For this review, take the finished solid that the model builds, in its own axes (mm). Face numbers are marked on the shaded views. A direction names the side the tool comes from. Round coordinates to 2 decimals unless told otherwise and drop trailing zeros. Order: outer loops, then holes, each group sorted by start corner. A loop starts at its lowest first (then second) coordinate and runs counter-clockwise, first axis right, second up. Notation, with made-up numbers: (-32.5, 36) -> (-3.5, 36) arc R20 ccw to (-3.5, 40) -> close; hole circle Ø4 at (-0.5, 70). An arc over 180 degrees is marked (long way). Answer in a Markdown table with one row per item.
```python
from build123d import *

# Parameters (mm, degrees)
F0_R     = 12.7
F0_R_2   = 6
F0_R_3   = 3.025
F1_DEPTH = 5
F2_DEPTH = 9
F3_D     = 2.4
F6_D     = 2.4
F6_DEPTH = 10
F6_TIP   = 0.7210327428


with BuildPart() as f1:
    # F0 (on Front) → F1 (new body)
    with BuildSketch(Plane.XZ):
        Circle(F0_R)
        Circle(F0_R_2, mode=Mode.SUBTRACT)
        Circle(F0_R_2)
        Circle(F0_R_3, mode=Mode.SUBTRACT)
    extrude(amount=F1_DEPTH)

    # F0 (on Front) → F2 (join)
    with BuildSketch(Plane.XZ):
        Circle(F0_R_2)
        Circle(F0_R_3, mode=Mode.SUBTRACT)
    extrude(amount=F2_DEPTH)

    # F3 (through all)
    with Locations(Plane(origin=(0, 0, 0), x_dir=(1, 0, 0), z_dir=(0, 1, 0))):
        with Locations((9.5, 0), (4.75, -8.227241336), (-4.75, -8.227241336), (-9.5, 0), (-4.75, 8.227241336), (4.75, 8.227241336)):
            Hole(F3_D / 2)

    # F6
    with Locations(Plane.XY.offset(12.7)):
        with Locations((0, -2.5), (0, -7)):
            Hole(F6_D / 2, depth=F6_DEPTH)
            with Locations((0, 0, -(F6_DEPTH + F6_TIP / 2))):  # 118° drill point
                Cone(0, F6_D / 2, F6_TIP, mode=Mode.SUBTRACT)


solid = f1.part
```
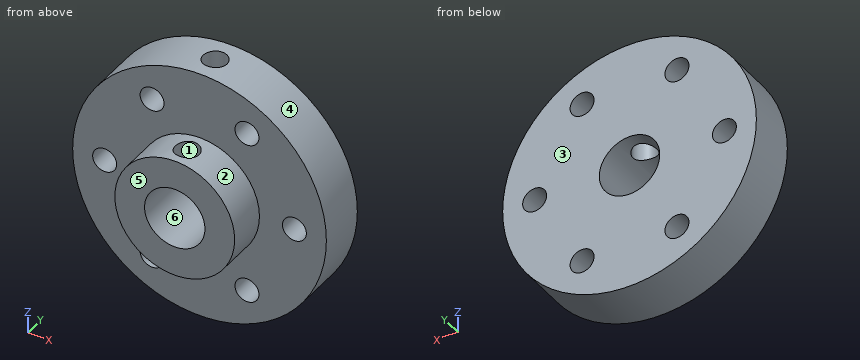
Q1. Take a section at C-C, the plane y = -1.75. Write out the cut boundary in (x, z) (3 decimals).
Answer key:
| item | result |
|---|---|
| outline | (-0.937, 2.876) -> (-0.937, 12.665) arc R12.7 ccw (long way) to (0.937, 12.665) -> (0.937, 2.876) arc R3.025 cw (long way) to start; hole circle Ø2.4 at (-9.5, 0); hole circle Ø2.4 at (-4.75, -8.227); hole circle Ø2.4 at (-4.75, 8.227); hole circle Ø2.4 at (4.75, -8.227); hole circle Ø2.4 at (4.75, 8.227); hole circle Ø2.4 at (9.5, 0) |
Q2. Take a section at D-D, the plane x = -4.25. Write out the cut boundary in (y, z), then the cut area to 3 significant figures.
Answer key:
| item | result |
|---|---|
| outline | (-9, -4.24) -> (-5, -4.24) -> (-5, -7.14) -> (0, -7.14) -> (0, 7.14) -> (-5, 7.14) -> (-5, 4.24) -> (-9, 4.24) -> close; (-5, -11.97) -> (0, -11.97) -> (0, -9.32) -> (-5, -9.32) -> close; (-5, 9.32) -> (0, 9.32) -> (0, 11.97) -> (-5, 11.97) -> close |
| area | 132 mm^2 |
Q3. Take a section at A-A, the plane x = 0. Write out the cut boundary in (y, z) (3 decimals).
Answer key:
| item | result |
|---|---|
| outline | (-9, -6) -> (-5, -6) -> (-5, -12.7) -> (0, -12.7) -> (0, -3.025) -> (-9, -3.025) -> close; (-9, 3.025) -> (-8.2, 3.025) -> (-8.2, 6) -> (-9, 6) -> close; (-5.8, 3.025) -> (-3.7, 3.025) -> (-3.7, 12.7) -> (-5, 12.7) -> (-5, 6) -> (-5.8, 6) -> close; (-1.3, 3.025) -> (0, 3.025) -> (0, 12.7) -> (-1.3, 12.7) -> close |
Q4. Clearance check with flat-ended pins moving along their axes: pin 1 Ø8 at (x, z) = (0, 0) entering from -Y; pin 2 Ø2 at (x, y) = (0, -7) entering from -Z; pin 3 Ø3 at (x, y) = (2.5, -5.5) entering from -Z; pin 4 Ø1.5 at (y, z) = (-3, -2) entering from -X. State where each tip first meets the part, or that it passes through.
Answer key:
| item | result |
|---|---|
| pin 1 | stops at y = -9 |
| pin 2 | stops at z = -6 |
| pin 3 | stops at z = -12.65 |
| pin 4 | stops at x = -12.64 |
Q5. To check wall thickness, follow probe 1 along Z at (x, y) = (4.75, -3.15); probe 2 along Y at (x, z) = (0, 8.5); probe 3 along X at (y, z) = (-0.5, 8.75). State the ranges of each line that lie inside material, in increasing order.
Answer key:
| item | result |
|---|---|
| probe 1 | z = -11.78 to -9.43, -7.03 to 7.03, 9.43 to 11.78 |
| probe 2 | y = -5 to -3.7, -1.3 to 0 |
| probe 3 | x = -9.2 to -5.83, -3.67 to 3.67, 5.83 to 9.2 |
Q6. Tool access review of the marked faces 1, 2 and 3: name each direction out of +Z, -Z, +X, -X, +Y, -Y from which nothing blocks a thin tool from reaching the whole face with its end or side.
Answer key:
| item | result |
|---|---|
| face 1 | +Z |
| face 2 | -Y |
| face 3 | +Z, -Z, +X, -X, +Y |
Q7. Take a section at B-B, the plane z = 2.25. Write out the cut boundary in (x, y), then the cut area to 3 significant figures.
Answer key:
| item | result |
|---|---|
| outline | (-12.5, -5) -> (-5.56, -5) -> (-5.56, -9) -> (-2.02, -9) -> (-2.02, 0) -> (-12.5, 0) -> close; (2.02, -9) -> (5.56, -9) -> (5.56, -5) -> (12.5, -5) -> (12.5, 0) -> (2.02, 0) -> close |
| area | 133 mm^2 |
Q8. The part is to be moulded in two halves that separate along Z. For the marked faces 4, 5 and 6, say which applies: +Z half, -Z half, draft (parallel to the pull), parting line (faces both ways), or undercut.
Answer key:
| item | result |
|---|---|
| face 4 | parting line |
| face 5 | draft |
| face 6 | undercut |
